from build123d import *

# Parameters (mm, degrees)
SKETCH1_W           = 29.4
SKETCH1_H           = 3
BOSS_EXTRUDE1_DEPTH = 3


with BuildPart() as part:
    # Sketch1 → Boss-Extrude1 (new body)
    with BuildSketch(Plane(origin=(0, 0, 0), x_dir=(1, 0, 0), z_dir=(0, 1, 0))):
        Polygon((-73.5, 7.5), (73.5, 7.5), (73.5, -15.5), (44.1, -15.5), (44.1, -12.5), (14.7, -12.5), (14.7, -15.5), (-14.7, -15.5), (-14.7, -12.5), (-44.1, -12.5), (-44.1, -15.5), (-73.5, -15.5), align=None)
        with Locations((29.4, 1)):
            Rectangle(SKETCH1_W, SKETCH1_H, mode=Mode.SUBTRACT)
        with Locations((-29.4, 1)):
            Rectangle(SKETCH1_W, SKETCH1_H, mode=Mode.SUBTRACT)
    extrude(amount=BOSS_EXTRUDE1_DEPTH)


solid = part.part
For this review, take the finished solid that the model builds, in its own axes (mm). A direction names the side the tool comes from. Give positions to 0.01 mm unless a question says otherwise; leave off trailing zeros. Order: outer loops, then holes, each group sorted by start corner. A loop starts at its lowest first (then second) coordinate and runs counter-clockwise, first axis right, second up. Notation, with made-up numbers: (53, 1.5) - (88, 1.5) arc R26 cw to (88, 24.5) - close; hole circle Ø10 at (55, -20.75). An arc over 180 degrees is marked (long way). Answer as a JSON object with one key per item and string values. Group by question number.
Item 1: Take a section at A-A on x = 42. Give the boundary of the cut face in (y, z).
Item 2: Draft analysis for pull direction X (two halves, no side actions). For faces 1 (the flat face through (-14.7, 1, 14)), 2 (the flat face through (-1, 1, -7.5)), 3 (the flat face through (-73.5, 1, 4)), 4 (the flat face through (73.5, 1, 4)), state which applies: pulls with the +X half, pulls with the -X half, needs draft (parallel to the pull), parting line crosses it, or undercut.
Item 3: Machinability: for faces 5 (the flat face through (29, 1, -2.5)), 6 (the flat face through (-59, 1, 15.5)), 7 (the flat face through (14.7, 1, 14)), which of the approach directions +Z, -Z, +X, -X, +Y, -Y give a long, thin tool a straight path to every point of the face, cutting with its end or side? Answer none if there is none.
Item 4: Wall thickness on line 1 along X through (y, z) = (0.5, 13.25); line 2 along Z through (x, y) = (44, 1.1): over which ranges is each line inside the solid? List them lowest first.
Item 5: Take a section at B-B on y = 1.65. Give the boundary of the cut face in (x, z), and give its area (3 significant figures).
Reported:
{
 "1": {"outline": "(0, -7.5) - (3, -7.5) - (3, -2.5) - (0, -2.5) - close; (0, 0.5) - (3, 0.5) - (3, 12.5) - (0, 12.5) - close"},
 "2": {"face 1": "undercut", "face 2": "needs draft", "face 3": "pulls with the -X half", "face 4": "pulls with the +X half"},
 "3": {"face 5": "+Y, -Y", "face 6": "+Z, +X, -X, +Y, -Y", "face 7": "+Z, +Y, -Y"},
 "4": {"line 1": "-73.5 to -44.1, -14.7 to 14.7, 44.1 to 73.5", "line 2": "-7.5 to -2.5, 0.5 to 12.5"},
 "5": {"outline": "(-73.5, -7.5) - (73.5, -7.5) - (73.5, 15.5) - (44.1, 15.5) - (44.1, 12.5) - (14.7, 12.5) - (14.7, 15.5) - (-14.7, 15.5) - (-14.7, 12.5) - (-44.1, 12.5) - (-44.1, 15.5) - (-73.5, 15.5) - close; hole (-44.1, -2.5) - (-14.7, -2.5) - (-14.7, 0.5) - (-44.1, 0.5) - close; hole (14.7, -2.5) - (44.1, -2.5) - (44.1, 0.5) - (14.7, 0.5) - close", "area": "3,030 mm^2"}
}
